Could you check a few things on this model? Use its own coordinates, in mm. A direction names the side the tool comes from. Round coordinates to 2 decimals unless told otherwise and drop trailing zeros. Order: outer loops, then holes, each group sorted by start corner. A loop starts at its lowest first (then second) coordinate and runs counter-clockwise, first axis right, second up. Notation, with made-up numbers: (77, 88.25) - (127, 88.25) arc R32 ccw to (127, 119.25) - close; hole circle Ø8 at (82.25, 45.25). An arc over 180 degrees is marked (long way). Use one line per item in the form item = value.
from build123d import *

# Parameters (mm, degrees)
SKETCH_1_R               = 50
EXTRUDE_1_DEPTH          = 6
SKETCH_2_R               = 35
EXTRUDE_2_DEPTH          = 60
SKETCH_4_W               = 77.448717432
SKETCH_4_H               = 33
CUT_EXTRUDE_2_DEPTH      = 40
SKETCH_5_W               = 12
SKETCH_5_H               = 45
CUT_EXTRUDE_3_DEPTH      = 30
CUT_EXTRUDE_4_DEPTH      = 97.726418315
CUT_EXTRUDE_4_DEPTH_BACK = 60
SKETCH_7_OUTSIDE_W       = 133.212
SKETCH_7_OUTSIDE_H       = 133.212
SKETCH_7_OUTSIDE_R       = 29.5
CUT_EXTRUDE_5_DEPTH      = 10
CUT_EXTRUDE_6_DEPTH      = 20
SKETCH_9_R               = 1.1
CUT_EXTRUDE_7_DEPTH      = 10
FILLET_1_R               = 2


with BuildPart() as part:
    # 草图1 → 凸台-拉伸1 (new body)
    with BuildSketch(Plane(origin=(0, 0, 0), x_dir=(1, 0, 0), z_dir=(0, 1, 0))):
        with Locations(Location((0, 0, 0), (0, 0, 270))):
            Circle(SKETCH_1_R)
    extrude(amount=EXTRUDE_1_DEPTH)

    # 草图2 → 凸台-拉伸2 (add)
    with BuildSketch(Plane.XZ):
        with Locations(Location((0, 0, 0), (0, 0, 270))):
            Circle(SKETCH_2_R)
    extrude(amount=EXTRUDE_2_DEPTH)

    # 草图4 → 切除-拉伸2 (cut)
    with BuildSketch(Plane.XZ.offset(60)):
        with Locations((2.029578549, -24.707284506)):
            Rectangle(SKETCH_4_W, SKETCH_4_H)
    extrude(amount=-CUT_EXTRUDE_2_DEPTH, mode=Mode.SUBTRACT)

    # 草图5 → 切除-拉伸3 (cut)
    with BuildSketch(Plane(origin=(0, 0, -8.207284506), x_dir=(-1, 0, 0), z_dir=(0, 0, -1))):
        with Locations((0, -42.5)):
            Rectangle(SKETCH_5_W, SKETCH_5_H)
    extrude(amount=-CUT_EXTRUDE_3_DEPTH, mode=Mode.SUBTRACT)

    # 草图6 → 切除-拉伸4 (cut, two sides: drawn at the far end of the back side and taken through both)
    with BuildSketch(Plane.XZ.offset(60).offset(-CUT_EXTRUDE_4_DEPTH_BACK)):
        with BuildLine():
            Line((-27.5, 0), (-25.651821524, -3.41877994))
            Line((-25.651821524, -3.41877994), (25.981995499, -3.41877994))
            Line((25.981995499, -3.41877994), (27.5, 0))
            ThreePointArc((27.5, 0), (0, 27.5), (-27.5, 0))
        make_face()
    extrude(amount=CUT_EXTRUDE_4_DEPTH + CUT_EXTRUDE_4_DEPTH_BACK, mode=Mode.SUBTRACT)

    # 草图7 outside → 切除-拉伸5 (cut)
    with BuildSketch(Plane.XZ.offset(60)):
        Rectangle(SKETCH_7_OUTSIDE_W, SKETCH_7_OUTSIDE_H)
        with Locations((0, 0.184250616)):
            Circle(SKETCH_7_OUTSIDE_R, mode=Mode.SUBTRACT)
    extrude(amount=-CUT_EXTRUDE_5_DEPTH, mode=Mode.SUBTRACT)

    # 草图8 → 切除-拉伸6 (cut)
    with BuildSketch(Plane.XZ.offset(20)):
        with BuildLine():
            Line((-29.384128464, -11.494001524), (28.615871536, -11.494001524))
            ThreePointArc((28.615871536, -11.494001524), (-0.384128464, -31.448176939), (-29.384128464, -11.494001524))
        make_face()
    extrude(amount=-CUT_EXTRUDE_6_DEPTH, mode=Mode.SUBTRACT)

    # 草图9 → 切除-拉伸7 (cut)
    with BuildSketch(Plane(origin=(0, 0, -8.207284506), x_dir=(-1, 0, 0), z_dir=(0, 0, -1))):
        with Locations((21.25, -28.140331005)):
            Circle(SKETCH_9_R)
        with Locations((21.25, -44.440331005)):
            Circle(SKETCH_9_R)
        with Locations((-21.25, -28.140331005)):
            Circle(SKETCH_9_R)
        with Locations((-21.25, -44.440331005)):
            Circle(SKETCH_9_R)
    extrude(amount=-CUT_EXTRUDE_7_DEPTH, mode=Mode.SUBTRACT)

    # 圆角1
    fillet_1_edges = [part.edges().sort_by_distance(p)[0] for p in [
        (-25.651821524, -30, -3.41877994),
        (27.5, -30, 0),
        (25.981995499, -30, -3.41877994),
        (-27.5, -30, 0),
    ]]
    fillet(fillet_1_edges, radius=FILLET_1_R)


solid = part.part
Item 1: Imagine slicing it at D-D on x = -16. Please give me the cut outline in (y, z), plus the area to 3 significant figures.
Found:
outline = (-60, -8.21) - (-20, -8.21) - (-20, -11.49) - (0, -11.49) - (0, -27.24) - (-20, -27.24) - (-20, -31.13) - (0, -31.13) - (0, -47.37) - (6, -47.37) - (6, 47.37) - (0, 47.37) - (0, 31.13) - (-50, 31.13) - (-50, 24.97) - (-60, 24.97) - (-60, 22.37) - (0, 22.37) - (0, -3.42) - (-60, -3.42) - close
area = 1,460 mm2
Item 2: For faces 5 (the face through (15.02, 2.96, 47.69)), 6 (the face through (0.641, -29.58, 27.493)), 7 (the face through (6, -40, -6)), 8 (the face through (20, -40, -8.207)), which set-ups out of +Z, -Z, +X, -X, +Y, -Y let a thin tool reach every point of the face, with its end or its side?
Found:
face_5 = +Y, -Y
face_6 = -Y
face_7 = -Z, -Y
face_8 = -Z, +X, -X, -Y
Item 3: Will these pins go through, and if not, where does the flat tip stop? P1, Ø15.5, axis at x = -1, z = 9, coming from the -Y side; P2, Ø6, axis at x = 0, y = -10.5, coming from the -Z side; P3, Ø22.5, axis at x = -17.5, y = -40.5, coming from the -Z side.
Found:
P1 = 0
P2 = -35
P3 = -8.21
Item 4: Imagine slicing it at B-B on y = -8. Please give me the cut outline in (x, z).
Found:
outline = circle Ø70 at (0, 0); hole (-29.38, -11.49) arc R31.05 ccw to (28.62, -11.49) - close; hole (-27.49, 0.54) arc R2 ccw to (-27.25, -0.45) - (-26.22, -2.37) arc R2 ccw to (-24.46, -3.42) - (24.68, -3.42) arc R2 ccw to (26.51, -2.23) - (27.32, -0.4) arc R2 ccw to (27.5, 0.45) arc R27.5 ccw to start
Item 5: I need wall thicknesses on L1, parallel to Y at x = 21.25, z = -5.3; L2, parallel to Y at x = 21, z = -5; L3, parallel to Z at x = -5.5, y = -15.5. Which ranges of each line are inside material? Lowest first, please.
Found:
L1 = -60 to -45.54, -43.34 to -29.24, -27.04 to 6
L2 = -60 to -45.51, -43.37 to -29.21, -27.07 to 6
L3 = -34.57 to -31.02, -11.49 to -3.42, 26.94 to 34.57
Item 6: Imagine slicing it at C-C on z = 24.5. Please give me the cut outline in (x, y) (3 decimals), plus the area to 3 significant figures.
Found:
outline = (-43.586, 0) - (-24.995, 0) - (-24.995, -50) - (-16.703, -50) - (-16.703, -60) - (-12.49, -60) - (-12.49, 0) - (12.49, 0) - (12.49, -60) - (16.703, -60) - (16.703, -50) - (24.995, -50) - (24.995, 0) - (43.586, 0) - (43.586, 6) - (-43.586, 6) - close
area = 1,860 mm2
Item 7: If we mould it in two halves opening along Z, with no side actions, what happens to faces 1 (the face through (-20, -40, -8.207)), 2 (the face through (-1, -10, -11.494)), 3 (the face through (1, 6, -1)), 4 (the face through (0, 0, -19))? For each: released by +Z, released by -Z, zero draft, split by the parting line, or undercut.
Found:
face_1 = released by -Z
face_2 = undercut
face_3 = zero draft
face_4 = undercut
Item 8: Imagine slicing it at A-A on y = -36. Please give me the cut outline in (x, z), plus the area to 3 significant figures.
Found:
outline = (-34.02, -8.21) - (-6, -8.21) - (-6, -3.42) - (-24.46, -3.42) arc R2 cw to (-26.22, -2.37) - (-27.25, -0.45) arc R2 cw to (-27.49, 0.54) arc R27.5 cw to (27.5, 0.45) arc R2 cw to (27.32, -0.4) - (26.51, -2.23) arc R2 cw to (24.68, -3.42) - (6, -3.42) - (6, -8.21) - (34.02, -8.21) arc R35 ccw (long way) to start
area = 1,070 mm2
